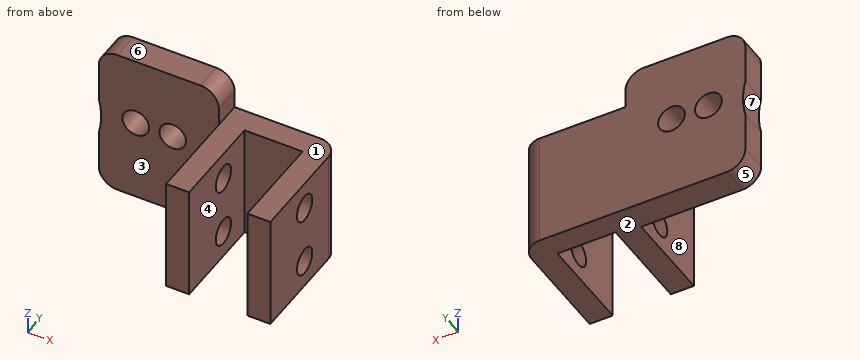
from build123d import *

# Parameters (mm, degrees)
F0_W      = 25
F0_H      = 3
F1_DEPTH  = 12.5
F2_W      = 25
F2_H      = 3
F3_DEPTH  = 4
F5_DEPTH  = 25
F6_DEPTH  = 15
F8_D      = 2.9
F9_DEPTH  = 25
F11_DEPTH = 25
F12_R     = 2
F13_D     = 2.9


with BuildPart() as f1:
    # F0 (on Top) → F1 (new body)
    with BuildSketch(Plane.XY):
        with Locations((-18.1500001341, 5.0000001341)):
            Rectangle(F0_W, F0_H)
        Polygon((3.15, 4), (3.15, -4), (3.15, -6.5000001341), (5.6500001341, -6.5000001341), (5.6500001341, 6.5000001341), (-5.6500001341, 6.5000001341), (-5.6500001341, 3.5000001341), (-5.6500001341, -6.5000001341), (-3.15, -6.5000001341), (-3.15, -4), (-3.15, 4), align=None)
    extrude(amount=F1_DEPTH)

    # F2 (on face) → F3 (join)
    with BuildSketch(Plane.XY.offset(12.5)):
        with Locations((-18.1500001341, 5.0000001341)):
            Rectangle(F2_W, F2_H)
    extrude(amount=F3_DEPTH)

    # F4 (on face) → F5 (cut)
    with BuildSketch(Plane(origin=(0, 6.5000001341, 0), x_dir=(-1, 0, 0), z_dir=(0, 1, 0))):
        with BuildLine():
            ThreePointArc((26.6500001341, 16.5), (28.7158126292, 16.2371721363), (30.6500001341, 15.4654348448))
            Line((30.6500001341, 15.4654348448), (30.6500001341, 16.5))
            Line((30.6500001341, 16.5), (26.6500001341, 16.5))
        make_face()
        with BuildLine():
            Line((30.6500001341, 0), (30.6500001341, 1.0345651552))
            ThreePointArc((30.6500001341, 1.0345651552), (28.7158126292, 0.2628278637), (26.6500001341, 0))
            Line((26.6500001341, 0), (30.6500001341, 0))
        make_face()
        with BuildLine():
            Line((30.6500001341, 6.1884471872), (30.6500001341, 10.3115528128))
            ThreePointArc((30.6500001341, 10.3115528128), (22.1500001341, 8.25), (30.6500001341, 6.1884471872))
        make_face()
    extrude(amount=-F5_DEPTH, mode=Mode.SUBTRACT)

    # F4 (on face) → F6 (join)
    with BuildSketch(Plane(origin=(0, 6.5000001341, 0), x_dir=(-1, 0, 0), z_dir=(0, 1, 0))):
        with BuildLine():
            ThreePointArc((30.6500001341, 6.1884471872), (22.1500001341, 8.25), (30.6500001341, 10.3115528128))
            Line((30.6500001341, 10.3115528128), (30.6500001341, 15.4654348448))
            ThreePointArc((30.6500001341, 15.4654348448), (28.7158126292, 16.2371721363), (26.6500001341, 16.5))
            ThreePointArc((26.6500001341, 16.5), (18.4000001341, 8.25), (26.6500001341, 0))
            ThreePointArc((26.6500001341, 0), (28.7158126292, 0.2628278637), (30.6500001341, 1.0345651552))
            Line((30.6500001341, 1.0345651552), (30.6500001341, 6.1884471872))
        make_face()
    extrude(amount=F6_DEPTH)

    # F8 (through all)
    with Locations(Plane.YZ.offset(5.6500001341)):
        with Locations((0.0002758615, 3), (0.0002758615, 9.5)):
            Hole(F8_D / 2)

    # F9 (cut): a face of the model
    f9_faces = [f1.faces().sort_by_distance(p)[0] for p in [
        (-30.444497701, 21.5000001341, 3.6115061712),
    ]]
    extrude(f9_faces, amount=-F9_DEPTH, mode=Mode.SUBTRACT)

    # F10 (on face) → F11 (cut)
    with BuildSketch(Plane(origin=(0, 6.5000001341, 0), x_dir=(-1, 0, 0), z_dir=(0, 1, 0))):
        with BuildLine():
            Line((18.6500001341, 16.5), (18.6500001341, 10.2655644371))
            ThreePointArc((18.6500001341, 10.2655644371), (21.5788023765, 14.7573384193), (26.6500001341, 16.5))
            Line((26.6500001341, 16.5), (18.6500001341, 16.5))
        make_face()
        with BuildLine():
            Line((18.6500001341, 6.2344355629), (18.6500001341, 0))
            Line((18.6500001341, 0), (26.6500001341, 0))
            ThreePointArc((26.6500001341, 0), (21.5788023765, 1.7426615807), (18.6500001341, 6.2344355629))
        make_face()
    extrude(amount=-F11_DEPTH, mode=Mode.SUBTRACT)

    # F12
    f12_edges = [f1.edges().sort_by_distance(p)[0] for p in [
        (-18.65, 5, 0),
        (-18.65, 5, 16.5),
        (-5.65, 5, 16.5),
        (5.65, 6.5, 6.25),
    ]]
    fillet(f12_edges, radius=F12_R)

    # F13 (through all)
    with Locations(Plane(origin=(0, 6.5000001341, 0), x_dir=(-1, 0, 0), z_dir=(0, 1, 0))):
        with Locations((14.6500001341, 9), (10.6500001341, 9)):
            Hole(F13_D / 2)


solid = f1.part
The listing builds one solid part. Answer for the finished solid, in the listing's coordinates (mm). Face numbers are marked on the shaded views. A direction names the side the tool comes from. Coordinates: 2 decimals unless noted, no trailing zeros. Order: outer loops, then holes, each group sorted by start corner. A loop starts at its lowest first (then second) coordinate and runs counter-clockwise, first axis right, second up. Notation, with made-up numbers: (-28.75, 15.5) -> (29.25, 15.5) arc R31 ccw to (29.25, 52.5) -> close; hole circle Ø7 at (31, 19.25). An arc over 180 degrees is marked (long way). Answer in a Markdown table with one row per item. Add a question column.
Item 1: Determine the mould class of the marked faces 5, 6, 7 and 8 for opening direction Z: +Z half, -Z half, draft (parallel to the pull), parting line (faces both ways), or undercut.
Item 2: Find section D-D (y = -0.5). Write down the section's boundary in (x, z).
Item 3: Find section A-A (z = 8.5). Write down the section's boundary in (x, y).
Item 4: Find section B-B (x = -10.65). Write down the section's boundary in (y, z), then the cut area to 3 significant figures.
Item 5: Each of these flat-tipped pins is pushed along its axis until it touches: P1, Ø3, axis at x = -5.5, y = -3, coming from the +Z side; P2, Ø5.5, axis at y = -2.5, z = 6, coming from the -X side; P3, Ø2.5, axis at x = -10.65, z = 9, coming from the +Y side; P4, Ø1.9, axis at x = -1, z = 4.5, coming from the -Y side. Where does it stop, or does it pass through?
Item 6: Which of the six approach directions +Z, -Z, +X, -X, +Y, -Y give full straight-line access (tool end or side, diameter ignored) to the marked faces 1, 2, 3 and 4?
Item 7: Find the intervals of material crossed by L1, parallel to X at y = -1.75, z = 8.5; L2, parallel to X at y = 6.25, z = 9.75; L3, parallel to Y at x = 2.25, z = 2.5, in increasing order. Write a range as from..to.
Item 8: Find section C-C (z = 3). Write down the section's boundary in (x, y), then the cut area to 3 significant figures.
Result set:
| question | item | result |
|---|---|---|
| 1 | face 5 | -Z half |
| 1 | face 6 | +Z half |
| 1 | face 7 | undercut |
| 1 | face 8 | draft |
| 2 | outline | (-5.65, 0) -> (-3.15, 0) -> (-3.15, 1.64) -> (-5.65, 1.64) -> close; (-5.65, 4.36) -> (-3.15, 4.36) -> (-3.15, 8.14) -> (-5.65, 8.14) -> close; (-5.65, 10.86) -> (-3.15, 10.86) -> (-3.15, 12.5) -> (-5.65, 12.5) -> close; (3.15, 0) -> (5.65, 0) -> (5.65, 1.64) -> (3.15, 1.64) -> close; (3.15, 4.36) -> (5.65, 4.36) -> (5.65, 8.14) -> (3.15, 8.14) -> close; (3.15, 10.86) -> (5.65, 10.86) -> (5.65, 12.5) -> (3.15, 12.5) -> close |
| 3 | outline | (-18.4, 3.5) -> (-16.01, 3.5) -> (-16.01, 6.5) -> (-18.4, 6.5) -> close; (-13.29, 3.5) -> (-12.01, 3.5) -> (-12.01, 6.5) -> (-13.29, 6.5) -> close; (-9.29, 3.5) -> (-5.65, 3.5) -> (-5.65, 1.05) -> (-3.15, 1.05) -> (-3.15, 4) -> (3.15, 4) -> (3.15, 1.05) -> (5.65, 1.05) -> (5.65, 4.5) arc R2 ccw to (3.65, 6.5) -> (-9.29, 6.5) -> close; (-5.65, -6.5) -> (-3.15, -6.5) -> (-3.15, -1.05) -> (-5.65, -1.05) -> close; (3.15, -6.5) -> (5.65, -6.5) -> (5.65, -1.05) -> (3.15, -1.05) -> close |
| 4 | outline | (3.5, 0) -> (6.5, 0) -> (6.5, 7.55) -> (3.5, 7.55) -> close; (3.5, 10.45) -> (6.5, 10.45) -> (6.5, 16.5) -> (3.5, 16.5) -> close |
| 4 | area | 40.8 mm² |
| 5 | P1 | stops at z = 12.5 |
| 5 | P2 | stops at x = -5.65 |
| 5 | P3 | passes through |
| 5 | P4 | stops at y = 4 |
| 6 | face 1 | +Z, +X, +Y, -Y |
| 6 | face 2 | -Z, +X, -X, +Y, -Y |
| 6 | face 3 | +Z, -Z, -X, -Y |
| 6 | face 4 | +Z, -Z, -Y |
| 7 | L1 | x = -5.65..-3.15, 3.15..5.65 |
| 7 | L2 | x = -18.54..-15.89, -13.41..-11.89, -9.41..4.62 |
| 7 | L3 | y = 4..6.5 |
| 8 | outline | (-18.65, 3.5) -> (-5.65, 3.5) -> (-5.65, 1.45) -> (-3.15, 1.45) -> (-3.15, 4) -> (3.15, 4) -> (3.15, 1.45) -> (5.65, 1.45) -> (5.65, 4.5) arc R2 ccw to (3.65, 6.5) -> (-18.65, 6.5) -> close; (-5.65, -6.5) -> (-3.15, -6.5) -> (-3.15, -1.45) -> (-5.65, -1.45) -> close; (3.15, -6.5) -> (5.65, -6.5) -> (5.65, -1.45) -> (3.15, -1.45) -> close |
| 8 | area | 104 mm² |
